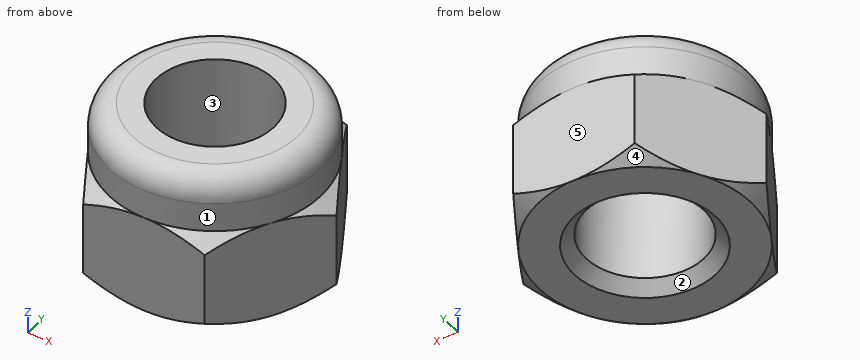
```python
from build123d import *

# Parameters (mm, degrees)
SKETCH1_R           = 1.5
BOSS_EXTRUDE1_DEPTH = 2.5
SKETCH2_R           = 2.69
SKETCH2_R_2         = 1.5
BOSS_EXTRUDE2_DEPTH = 1.34
FILLET1_R           = 0.6
CHAMFER1_SIZE       = 0.3


with BuildPart() as part:
    # Sketch1 → Boss-Extrude1 (new body)
    with BuildSketch(Plane.XY):
        Polygon((-1.553072224, 2.69), (1.553072224, 2.69), (3.106144448, 0), (1.553072224, -2.69), (-1.553072224, -2.69), (-3.106144448, 0), align=None)
        Circle(SKETCH1_R, mode=Mode.SUBTRACT)
    extrude(amount=BOSS_EXTRUDE1_DEPTH)

    # Sketch2 → Boss-Extrude2 (add)
    with BuildSketch(Plane.XY.offset(2.5)):
        Circle(SKETCH2_R)
        Circle(SKETCH2_R_2, mode=Mode.SUBTRACT)
    extrude(amount=BOSS_EXTRUDE2_DEPTH)

    # Fillet1
    fillet1_edges = [part.edges().sort_by_distance(p)[0] for p in [
        (-2.69, 0, 3.84),
    ]]
    fillet(fillet1_edges, radius=FILLET1_R)

    # Sketch3 → Cut-Revolve1 (revolve, cut)
    with BuildSketch(Plane(origin=(0, 0, 0), x_dir=(0, 0, -1), z_dir=(1, 0, 0))):
        Polygon((-2.5, 2.69), (-2.109788941, 3.19), (-0.390211059, 3.19), (0, 2.69), (0, 3.325081684), (-2.5, 3.325081684), align=None)
    revolve(axis=Axis((0, 0, 0), (0, 0, -1)), mode=Mode.SUBTRACT)

    # Chamfer1
    chamfer1_edges = [part.edges().sort_by_distance(p)[0] for p in [
        (-1.5, 0, 0),
    ]]
    chamfer(chamfer1_edges, length=CHAMFER1_SIZE)


solid = part.part
```
Can you work these out from the model? Positions are in its coordinate system, mm. Face numbers are marked on the shaded views. A direction names the side the tool comes from. Coordinates: 2 decimals unless noted, no trailing zeros. Order: outer loops, then holes, each group sorted by start corner. A loop starts at its lowest first (then second) coordinate and runs counter-clockwise, first axis right, second up.
1. If we section it at B-B (z = 2.9): Please give me the cut outline in (x, y), then the cut area to 3 significant figures.
2. I need wall thicknesses on line 1 (Y direction, x = 0, z = 3.15); line 2 (X direction, y = -1.25, z = 3.4); line 3 (X direction, y = 0.2, z = 1.8). Which ranges of each line are inside material? Lowest first, please.
3. For the marked faces 1 and 2, which set-ups out of +Z, -Z, +X, -X, +Y, -Y let a thin tool reach every point of the face, with its end or its side?
4. If we section it at A-A (z = 0.95): Please give me the cut outline in (x, y).
5. Thinking about a two-plate mould opening in X: for the marked faces 3, 4 and 5, which applies, +X half, -X half, draft (parallel to the pull), parting line (faces both ways), or undercut?
Entries:
1. outline: circle Ø5.38 at (0, 0); hole circle Ø3 at (0, 0)
1. area: 15.7 mm2
2. line 1: y = -2.69 to -1.5, 1.5 to 2.69
2. line 2: x = -2.36 to -0.83, 0.83 to 2.36
2. line 3: x = -2.99 to -1.49, 1.49 to 2.99
3. face 1: +Z
3. face 2: -Z
4. outline: (-3.11, 0) - (-1.55, -2.69) - (1.55, -2.69) - (3.11, 0) - (1.55, 2.69) - (-1.55, 2.69) - close; hole circle Ø3 at (0, 0)
5. face 3: undercut
5. face 4: -X half
5. face 5: draft
